The drawing under review shows one solid part. Ordinate dimensions are in mm from its lowest x, y, z. A direction names the side the tool comes from. Round coordinates to 2 decimals unless told otherwise and drop trailing zeros. Write each loop counter-clockwise with the first axis right and the second up, starting at its lowest first coordinate (ties: lowest second). Pieces come first, ordered by that corner, then holes. Notation, with made-up numbers: (64.25, 35.5) -> (121.25, 35.5) arc R8 ccw to (121.25, 43.5) -> close; hole circle Ø7 at (16, 28). An arc over 180 degrees is marked (long way). Answer in a Markdown table with one row per item. Add a question column.
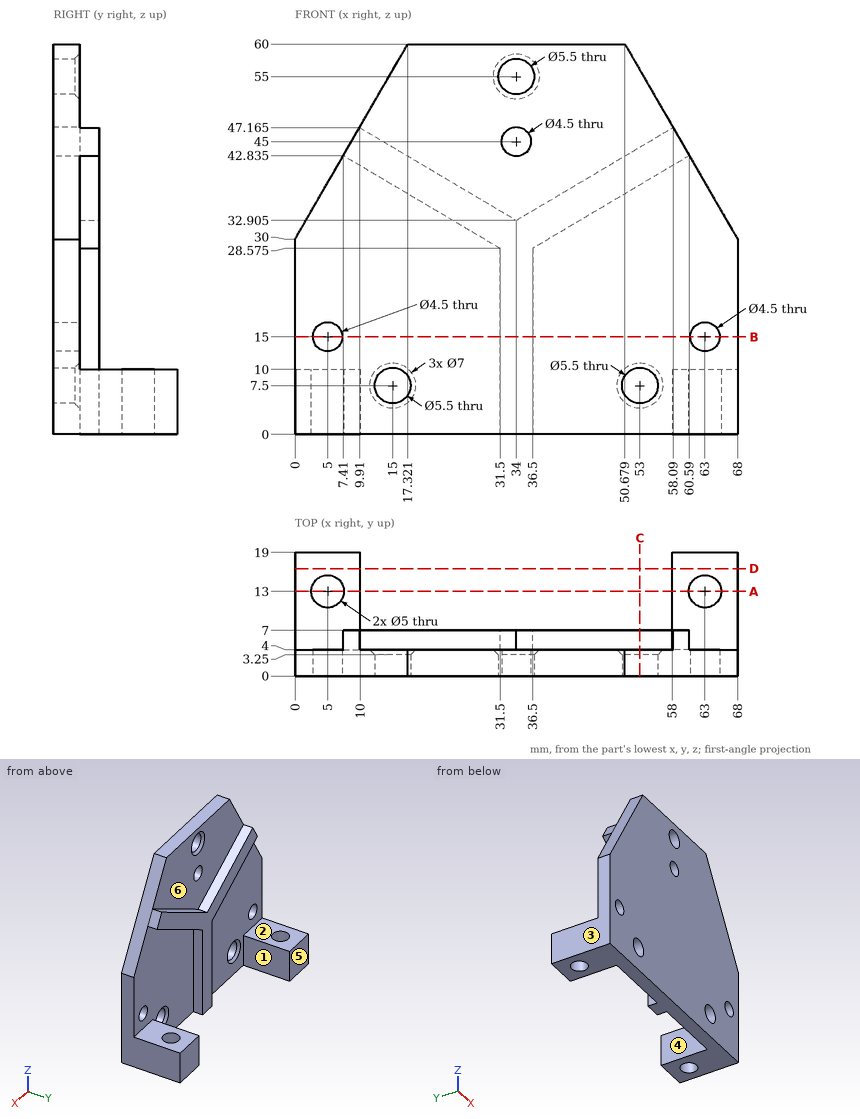
1. Add section C-C on x = 53. Write out the cut boundary in (y, z).
2. Add section D-D on y = 16.5. Write out the cut boundary in (x, z).
3. Add section A-A on y = 13. Write out the cut boundary in (x, z).
4. For L1, parallel to X at y = 2, z = 7.5; L2, parallel to X at y = 6.5, z = 5.5; L3, parallel to Y at x = 5, z = 5.5, list the stretches that pass through material, from the lowest coordinate up.
5. Insertion check: pin 1 Ø2.5 at (y, z) = (5.5, 16) entering from -X; pin 2 Ø8 at (x, z) = (26, 48.5) entering from +Y; pin 3 Ø3 at (x, y) = (6.5, 14.5) entering from +Z. Each pin has a flat end and moves straight along its axis. Give the tip position at first contact, or say it passes through.
6. Mouldability with a two-part tool opening along X and no side actions: class the marked faces 1, 2, 3 and 4 as pulls with the +X half, pulls with the -X half, needs draft (parallel to the pull), parting line crosses it, or undercut.
7. Add section B-B on z = 15. Write out the cut boundary in (x, y), plus the area to 3 significant figures.
8. Tool access review of the marked faces 5 and 6: name each direction out of +Z, -Z, +X, -X, +Y, -Y from which nothing blocks a thin tool from reaching the whole face with its end or side.
Filled in:
| question | item | result |
|---|---|---|
| 1 | outline | (0, 0) -> (4, 0) -> (4, 4) -> (3.25, 4.75) -> (0, 4.75) -> close; (0, 10.25) -> (3.25, 10.25) -> (4, 11) -> (4, 38.34) -> (7, 38.34) -> (7, 44.15) -> (4, 44.15) -> (4, 55.98) -> (0, 55.98) -> close |
| 2 | outline | (0, 0) -> (10, 0) -> (10, 10) -> (0, 10) -> close; (58, 0) -> (68, 0) -> (68, 10) -> (58, 10) -> close |
| 3 | outline | (0, 0) -> (2.5, 0) -> (2.5, 10) -> (0, 10) -> close; (7.5, 0) -> (10, 0) -> (10, 10) -> (7.5, 10) -> close; (58, 0) -> (60.5, 0) -> (60.5, 10) -> (58, 10) -> close; (65.5, 0) -> (68, 0) -> (68, 10) -> (65.5, 10) -> close |
| 4 | L1 | 0 to 12.25, 17.75 to 50.25, 55.75 to 68 |
| 4 | L2 | 0 to 10, 31.5 to 36.5, 58 to 68 |
| 4 | L3 | 0 to 10.5, 15.5 to 19 |
| 5 | pin 1 | x = 31.5 |
| 5 | pin 2 | y = 4 |
| 5 | pin 3 | z = 10 |
| 6 | face 1 | undercut |
| 6 | face 2 | needs draft |
| 6 | face 3 | pulls with the -X half |
| 6 | face 4 | undercut |
| 7 | outline | (0, 0) -> (2.75, 0) -> (2.75, 4) -> (0, 4) -> close; (7.25, 0) -> (60.75, 0) -> (60.75, 4) -> (36.5, 4) -> (36.5, 7) -> (31.5, 7) -> (31.5, 4) -> (7.25, 4) -> close; (65.25, 0) -> (68, 0) -> (68, 4) -> (65.25, 4) -> close |
| 7 | area | 251 mm² |
| 8 | face 5 | +Z, -Z, +X, -X, +Y |
| 8 | face 6 | +Z, +Y |
